from build123d import *

# Parameters (mm, degrees)
SKETCH1_W           = 3
SKETCH1_H           = 30
SKETCH1_W_2         = 10
SKETCH1_H_2         = 3
BOSS_EXTRUDE2_DEPTH = 1.5


with BuildPart() as part:
    # Sketch1 → Boss-Extrude2 (new body, symmetric)
    with BuildSketch(Plane.XY):
        Polygon((10, 40), (15, 40), (15, 0), (35, 0), (35, -40), (20, -40), (20, -43), (0, -43), (0, -40), (-15, -40), (-15, 40), (-10, 40), (-10, 43), (10, 43), align=None)
        with Locations((-12.5, 0)):
            Rectangle(SKETCH1_W, SKETCH1_H, mode=Mode.SUBTRACT)
        with Locations((12.5, 0)):
            Rectangle(SKETCH1_W, SKETCH1_H, mode=Mode.SUBTRACT)
        with Locations((25, -3.5)):
            Rectangle(SKETCH1_W_2, SKETCH1_H_2, mode=Mode.SUBTRACT)
    extrude(amount=BOSS_EXTRUDE2_DEPTH, both=True)


solid = part.part
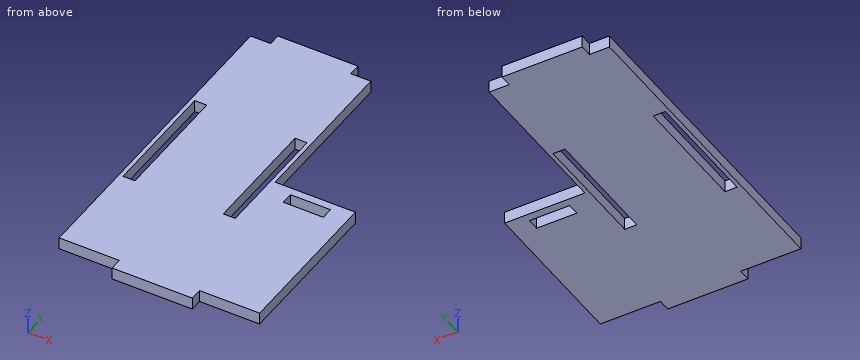
Build history of the part. All positions in model axes, mm. Coordinates: 2 decimals unless noted, no trailing zeros. Write each loop counter-clockwise with the first axis right and the second up, starting at its lowest first coordinate (ties: lowest second). Pieces come first, ordered by that corner, then holes.
(1) Pin check, flat tips, straight feed: pin 1 Ø5 at (x, y) = (25, 0.5) entering from -Z; pin 2 Ø1.5 at (x, z) = (-12.5, 0.5) entering from +Y; pin 3 Ø1.5 at (y, z) = (-41, 0) entering from -X; pin 4 Ø0.9 at (x, z) = (-13, -0.5) entering from -Y. Stop position of each tip, or through.
(2) Cut at D-D on y = -9.5. List the corners of the cut face in (x, z), and give its area (3 significant figures).
(3) Cut at A-A on x = 27.5. List the corners of the cut face in (y, z), and give its area (3 significant figures).
(4) Drill centre lines: line 1 (X direction, y = -7, z = -0.7); line 2 (X direction, y = 11.5, z = -0.5); line 3 (Y direction, x = 24, z = -0.85). Where is each one in solid material? Low to high.
(5) Cut at B-B on y = 10.5. List the corners of the cut face in (x, z), and give its area (3 significant figures).
(6) Cut at C-C on z = -0.05. List the corners of the cut face in (x, y).
Working result:
1. pin 1: stops at z = -1.5
1. pin 2: stops at y = 40
1. pin 3: stops at x = 0
1. pin 4: stops at y = -40
2. outline: (-15, -1.5) - (-14, -1.5) - (-14, 1.5) - (-15, 1.5) - close; (-11, -1.5) - (11, -1.5) - (11, 1.5) - (-11, 1.5) - close; (14, -1.5) - (35, -1.5) - (35, 1.5) - (14, 1.5) - close
2. area: 132 mm2
3. outline: (-40, -1.5) - (-5, -1.5) - (-5, 1.5) - (-40, 1.5) - close; (-2, -1.5) - (0, -1.5) - (0, 1.5) - (-2, 1.5) - close
3. area: 111 mm2
4. line 1: x = -15 to -14, -11 to 11, 14 to 35
4. line 2: x = -15 to -14, -11 to 11, 14 to 15
4. line 3: y = -40 to -5, -2 to 0
5. outline: (-15, -1.5) - (-14, -1.5) - (-14, 1.5) - (-15, 1.5) - close; (-11, -1.5) - (11, -1.5) - (11, 1.5) - (-11, 1.5) - close; (14, -1.5) - (15, -1.5) - (15, 1.5) - (14, 1.5) - close
5. area: 72.0 mm2
6. outline: (-15, -40) - (0, -40) - (0, -43) - (20, -43) - (20, -40) - (35, -40) - (35, 0) - (15, 0) - (15, 40) - (10, 40) - (10, 43) - (-10, 43) - (-10, 40) - (-15, 40) - close; hole (-14, -15) - (-11, -15) - (-11, 15) - (-14, 15) - close; hole (11, -15) - (14, -15) - (14, 15) - (11, 15) - close; hole (20, -5) - (30, -5) - (30, -2) - (20, -2) - close
